```python
from build123d import *

# Parameters (mm, degrees)
SKETCH_3_W          = 66
SKETCH_3_H          = 60
EXTRUDE_1_DEPTH     = 3
SKETCH_1_W          = 3.5
SKETCH_1_H          = 10.5
SKETCH_1_W_2        = 10.5
SKETCH_1_H_2        = 3.5
SKETCH_1_H_3        = 9.75
SKETCH_1_H_4        = 4.5
CUT_EXTRUDE_1_DEPTH = 49.597691494


with BuildPart() as part:
    # Эскиз3 → Бобышка-Вытянуть1 (new body)
    with BuildSketch(Plane(origin=(0, 0, 0), x_dir=(1, 0, 0), z_dir=(0, 1, 0))):
        with Locations((0, 5.54905932)):
            Rectangle(SKETCH_3_W, SKETCH_3_H)
    extrude(amount=EXTRUDE_1_DEPTH)

    # Эскиз1 → Вырез-Вытянуть1 (cut, through all)
    with BuildSketch(Plane(origin=(0, 0, 0), x_dir=(1, 0, 0), z_dir=(0, 1, 0))):
        with Locations((-29, 5.54905932)):
            Rectangle(SKETCH_1_W, SKETCH_1_H)
        with Locations((-29, 20.54905932)):
            Rectangle(SKETCH_1_W, SKETCH_1_H)
        with Locations((-29, -9.45094068)):
            Rectangle(SKETCH_1_W, SKETCH_1_H)
        with Locations((12.5, 21.54905932)):
            Rectangle(SKETCH_1_W_2, SKETCH_1_H_2)
        with Locations((29, -19.57594068)):
            Rectangle(SKETCH_1_W, SKETCH_1_H_3)
        with Locations((29, 13.04905932)):
            Rectangle(SKETCH_1_W, SKETCH_1_H_4)
        with Locations((29, -1.95094068)):
            Rectangle(SKETCH_1_W, SKETCH_1_H_4)
        with Locations((29, 30.67405932)):
            Rectangle(SKETCH_1_W, SKETCH_1_H_3)
        with Locations((-12.5, 21.54905932)):
            Rectangle(SKETCH_1_W_2, SKETCH_1_H_2)
    extrude(amount=CUT_EXTRUDE_1_DEPTH, mode=Mode.SUBTRACT)


solid = part.part
```
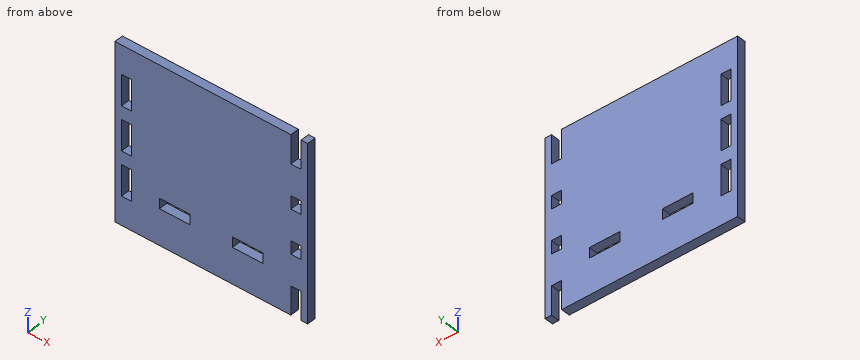
The model under review builds one solid part; all positions refer to its coordinate system, in mm. Coordinates: 2 decimals unless noted, no trailing zeros. Write each loop counter-clockwise with the first axis right and the second up, starting at its lowest first coordinate (ties: lowest second). Pieces come first, ordered by that corner, then holes. Notation, with made-up numbers: (30, 0) - (52, 0) arc R18 cw to (52, 18) - close; hole circle Ø1 at (-28, 45.25). An arc over 180 degrees is marked (long way). Answer in a Markdown table with one row per item. Add a question column.
Q1. Consider section D-D on y = 1.6. Give the number of separate pieces and of enclosed holes in the cut face, then the cut area to 3 significant figures.
Q2. Consider section B-B on x = 11.5. Give the boundary of the cut face in (y, z).
Q3. To check wall thickness, follow line 1 along Z through (x, y) = (-30, 0.9); line 2 along X through (y, z) = (0.2, 9); line 3 along Z through (x, y) = (11, 0.95). State the ranges of each line that lie inside material, in increasing order. Write a range as from..to.
Q4. Consider section A-A on z = -22. Give the boundary of the cut face in (x, y).
Q5. Clearance check with a flat-ended pin moving along its axis: pin 1 (1.5 mm diameter, centred on x = 29.5, y = 2, fed in from +Z). State where the tip first meets the part, or that it passes through.
Q6. Consider section C-C on z = 1.5. Give the boundary of the cut face in (x, y), then the cut area to 4 significant figures.
Answers below:
| question | item | result |
|---|---|---|
| 1 | separate pieces | 1 |
| 1 | enclosed holes | 7 |
| 1 | area | 3,680 mm² |
| 2 | outline | (0, -35.55) - (3, -35.55) - (3, -23.3) - (0, -23.3) - close; (0, -19.8) - (3, -19.8) - (3, 24.45) - (0, 24.45) - close |
| 3 | line 1 | -35.55..-25.8, -15.3..-10.8, -0.3..4.2, 14.7..24.45 |
| 3 | line 2 | -33..-30.75, -27.25..33 |
| 3 | line 3 | -35.55..-23.3, -19.8..24.45 |
| 4 | outline | (-33, 0) - (-30.75, 0) - (-30.75, 3) - (-33, 3) - close; (-27.25, 0) - (-17.75, 0) - (-17.75, 3) - (-27.25, 3) - close; (-7.25, 0) - (7.25, 0) - (7.25, 3) - (-7.25, 3) - close; (17.75, 0) - (33, 0) - (33, 3) - (17.75, 3) - close |
| 5 | pin 1 | z = 14.7 |
| 6 | outline | (-33, 0) - (27.25, 0) - (27.25, 3) - (-33, 3) - close; (30.75, 0) - (33, 0) - (33, 3) - (30.75, 3) - close |
| 6 | area | 187.5 mm² |
